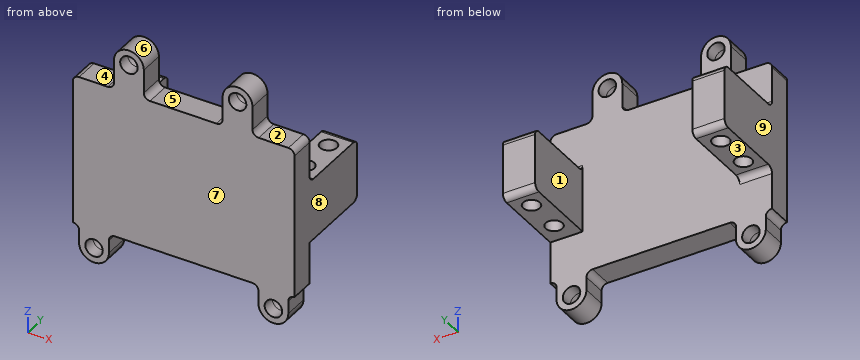
```python
from build123d import *
from build123d.topology import SkipClean

# Parameters (mm, degrees)
SKETCH1_W           = 54.4
SKETCH1_H           = 38.8
BOSS_EXTRUDE1_DEPTH = 3.175
SKETCH2_W           = 7
SKETCH2_H           = 15.875
BOSS_EXTRUDE2_DEPTH = 20
SKETCH3_R           = 3.8354
SKETCH3_R_2         = 2.2479
BOSS_EXTRUDE3_DEPTH = 3.175
LPATTERN1_COUNT     = 2
LPATTERN1_PITCH     = 27.94
SKETCH6_R           = 3.8354
SKETCH6_R_2         = 2.2479
BOSS_EXTRUDE6_DEPTH = 3.175
SKETCH7_R           = 2.150000018
CUT_EXTRUDE1_DEPTH  = 15.875
BOSS_EXTRUDE7_DEPTH = 1.2948
SKETCH11_R          = 2.2479
BOSS_EXTRUDE8_DEPTH = 3.175
FILLET1_R           = 1.5875


with BuildPart() as part:
    # Sketch1 → Boss-Extrude1 (new body)
    with BuildSketch(Plane(origin=(0, 0, 0), x_dir=(1, 0, 0), z_dir=(0, 1, 0))):
        with Locations((27.2, 19.4)):
            Rectangle(SKETCH1_W, SKETCH1_H)
    extrude(amount=BOSS_EXTRUDE1_DEPTH)

    # Sketch2 → Boss-Extrude2 (add)
    with BuildSketch(Plane(origin=(0, 3.175, 0), x_dir=(1, 0, 0), z_dir=(0, 1, 0))):
        with Locations((3.5, 20.0625)):
            Rectangle(SKETCH2_W, SKETCH2_H)
    boss_extrude2 = extrude(amount=BOSS_EXTRUDE2_DEPTH)

    # Mirror1: Boss-Extrude2 across plane
    add(boss_extrude2.mirror(Plane.ZY.offset(-27.2)))

    # Sketch3 → Boss-Extrude3 (add)
    # profile 1 of 2: a face of its own
    with BuildSketch(Plane(origin=(0, 3.175, 0), x_dir=(1, 0, 0), z_dir=(0, 1, 0))):
        with Locations((13.109999942, -7.608)):
            Circle(SKETCH3_R)
        with Locations(Location((13.109999942, -7.608, 0), (0, 0, 270))):
            Circle(SKETCH3_R_2, mode=Mode.SUBTRACT)
    # profile 2 of 2: a face of its own
    with BuildSketch(Plane(origin=(0, 3.175, 0), x_dir=(1, 0, 0), z_dir=(0, 1, 0))):
        with BuildLine():
            Line((9.274599942, 0), (9.274599942, -7.608))
            ThreePointArc((9.274599942, -7.608), (13.109999942, -3.7726), (16.945399942, -7.608))
            Line((16.945399942, -7.608), (16.945399942, 0))
            Line((16.945399942, 0), (9.274599942, 0))
        make_face()
    boss_extrude3 = extrude(amount=-BOSS_EXTRUDE3_DEPTH)

    # LPattern1: Boss-Extrude3 ×2
    with Locations(*[(i * LPATTERN1_PITCH, 0, 0) for i in range(1, LPATTERN1_COUNT)]):
        add(boss_extrude3)

    # Sketch6 → Boss-Extrude6 (add)
    # profile 1 of 2: a face of its own
    with BuildSketch(Plane(origin=(0, 3.175, 0), x_dir=(1, 0, 0), z_dir=(0, 1, 0))):
        with Locations((4.1402, 43.7)):
            Circle(SKETCH6_R)
        with Locations(Location((4.1402, 43.7, 0), (0, 0, 270))):
            Circle(SKETCH6_R_2, mode=Mode.SUBTRACT)
    # profile 2 of 2: a face of its own
    with BuildSketch(Plane(origin=(0, 3.175, 0), x_dir=(1, 0, 0), z_dir=(0, 1, 0))):
        with BuildLine():
            ThreePointArc((7.9756, 43.7), (4.1402, 39.8646), (0.3048, 43.7))
            Line((0.3048, 43.7), (0.3048, 38.8))
            Line((0.3048, 38.8), (7.9756, 38.8))
            Line((7.9756, 38.8), (7.9756, 43.7))
        make_face()
    boss_extrude6 = extrude(amount=-BOSS_EXTRUDE6_DEPTH)

    # Mirror3: Boss-Extrude6 across plane
    add(boss_extrude6.mirror(Plane.ZY.offset(-27.2)))

    # Sketch7 → Cut-Extrude1 (cut)
    with BuildSketch(Plane(origin=(0, 0, -28), x_dir=(-1, 0, 0), z_dir=(0, 0, -1))):
        with Locations((-2.852600116, 17.925)):
            Circle(SKETCH7_R)
        with Locations((-2.852600116, 8.425)):
            Circle(SKETCH7_R)
    cut_extrude1 = extrude(amount=-CUT_EXTRUDE1_DEPTH, mode=Mode.SUBTRACT)

    # Sketch9 → Boss-Extrude7 (add)
    with BuildSketch(Plane.ZY):
        Polygon((-38.8, 0), (-38.8, 3.175), (-28, 3.175), (-28, 23.175), (-12.125, 23.175), (-12.125, 3.175), (0, 3.175), (0, 0), align=None)
    boss_extrude7 = extrude(amount=BOSS_EXTRUDE7_DEPTH)

    # Mirror4: Boss-Extrude7 across plane
    add(boss_extrude7.mirror(Plane.ZY.offset(-27.2)))

    # Mirror5: Cut-Extrude1 across plane
    add(cut_extrude1.mirror(Plane.ZY.offset(-27.2)), mode=Mode.SUBTRACT)

    # Sketch11 → Boss-Extrude8 (add)
    with SkipClean():  # the faces are left unmerged after this step: merging them gives an invalid solid
        with BuildSketch(Plane.XZ):
            with BuildLine():
                Line((0.3048, -38.8), (0.3048, -43.7))
                ThreePointArc((0.3048, -43.7), (4.1402, -47.5354), (7.9756, -43.7))
                Line((7.9756, -43.7), (7.9756, -38.8))
                Line((7.9756, -38.8), (46.4244, -38.8))
                Line((46.4244, -38.8), (46.4244, -43.7))
                ThreePointArc((46.4244, -43.7), (50.2598, -47.5354), (54.0952, -43.7))
                Line((54.0952, -43.7), (54.0952, -38.8))
                Line((54.0952, -38.8), (55.6948, -38.8))
                Line((55.6948, -38.8), (55.6948, 0))
                Line((55.6948, 0), (44.885399942, 0))
                Line((44.885399942, 0), (44.885399942, 7.608))
                ThreePointArc((44.885399942, 7.608), (41.049999942, 11.4434), (37.214599942, 7.608))
                Line((37.214599942, 7.608), (37.214599942, 0))
                Line((37.214599942, 0), (16.945399942, 0))
                Line((16.945399942, 0), (16.945399942, 7.608))
                ThreePointArc((16.945399942, 7.608), (13.109999942, 11.4434), (9.274599942, 7.608))
                Line((9.274599942, 7.608), (9.274599942, 0))
                Line((9.274599942, 0), (-1.2948, 0))
                Line((-1.2948, 0), (-1.2948, -38.8))
                Line((-1.2948, -38.8), (0.3048, -38.8))
            make_face()
            with Locations(Location((4.1402, -43.7, 0), (0, 0, 90))):
                Circle(SKETCH11_R, mode=Mode.SUBTRACT)
            with Locations(Location((50.2598, -43.7, 0), (0, 0, 90))):
                Circle(SKETCH11_R, mode=Mode.SUBTRACT)
            with Locations(Location((41.049999942, 7.608, 0), (0, 0, 90))):
                Circle(SKETCH11_R, mode=Mode.SUBTRACT)
            with Locations(Location((13.109999942, 7.608, 0), (0, 0, 90))):
                Circle(SKETCH11_R, mode=Mode.SUBTRACT)
        extrude(amount=BOSS_EXTRUDE8_DEPTH)
    add(part.part.scale(1), mode=Mode.REPLACE)  # the faces are merged on a copy

    # Fillet1
    fillet1_edges = [part.edges().sort_by_distance(p)[0] for p in [
        (-1.2948, 0, 0),
        (55.6948, 0, 0),
        (2.8526, 3.175, -12.125),
        (2.8526, 3.175, -28),
        (2.8526, 23.175, -12.125),
        (2.8526, 23.175, -28),
        (51.5474, 23.175, -28),
        (51.5474, 23.175, -12.125),
        (51.5474, 3.175, -12.125),
        (16.945399942, 0, 0),
        (9.274599942, 0, 0),
        (44.885399942, 0, 0),
        (37.214599942, 0, 0),
        (0.3048, 0, -38.8),
        (7.9756, 0, -38.8),
        (46.4244, 0, -38.8),
        (54.0952, 0, -38.8),
    ]]
    fillet(fillet1_edges, radius=FILLET1_R)


solid = part.part
```
Read the model definition and answer for the solid it produces. Units are mm, in the model's axes. Face numbers are marked on the shaded views. A direction names the side the tool comes from. Give positions to 0.01 mm unless a question says otherwise; leave off trailing zeros. Loops run counter-clockwise (first coordinate to the right, second up) from the corner with the lowest first, then second, coordinate; pieces in that order, holes last.
Item 1: Find the intervals of material crossed by line 1 along Z through (x, y) = (13.11, 1.3); line 2 along X through (y, z) = (20.75, -20.5); line 3 along X through (y, z) = (0.25, 7.5), in increasing order.
Item 2: The mould has two halves that part along X. Classify the marked faces 6, 7, 8 and 9: released by +X, released by -X, zero draft, split by the parting line, or undercut.
Item 3: The part is cut by section C-C (x = 13.11). Write down the section's boundary in (y, z) (3 decimals).
Item 4: The part is cut by section B-B (y = 19.25). Write down the section's boundary in (x, z) (3 decimals), and give its area (3 significant figures).
Item 5: Each of these flat-tipped pins is pushed along its axis until it touches: pin 1 Ø2.5 at (x, y) = (52, 16.5) entering from -Z; pin 2 Ø3.5 at (x, y) = (51.55, 8.43) entering from -Z; pin 3 Ø4 at (x, y) = (51, 16.5) entering from +Z (3 decimals); pin 4 Ø1 at (y, z) = (0.5, -43) entering from -X. Where does it stop, or does it pass through?
Item 6: For the marked faces 1, 2, 3, 4 and 5, determine the directions among +Z, -Z, +X, -X, +Y, -Y from which every point of the face is accessible in a straight line to the end or side of a thin tool.
Item 7: The part is cut by section D-D (y = -1.5). Give the number of separate pieces and of enclosed holes in the cut face, and give its area (3 significant figures).
Item 8: The part is cut by section A-A (z = 4). Write down the section's boundary in (x, y) (3 decimals).
Taken from the geometry:
1. line 1: z = -38.8 to 5.36, 9.86 to 11.44
1. line 2: x = -1.29 to 7, 47.4 to 55.69
1. line 3: x = 9.27 to 10.86, 15.36 to 16.95, 37.21 to 38.8, 43.3 to 44.89
2. face 6: undercut
2. face 7: zero draft
2. face 8: released by +X
2. face 9: released by -X
3. outline: (-3.175, -38.8) - (3.175, -38.8) - (3.175, 5.36) - (-3.175, 5.36) - close; (-3.175, 9.856) - (3.175, 9.856) - (3.175, 11.443) - (-3.175, 11.443) - close
4. outline: (-1.295, -28) - (1.159, -28) - (1.159, -12.125) - (-1.295, -12.125) - close; (4.546, -28) - (7, -28) - (7, -12.125) - (4.546, -12.125) - close; (47.4, -28) - (49.854, -28) - (49.854, -12.125) - (47.4, -12.125) - close; (53.241, -28) - (55.695, -28) - (55.695, -12.125) - (53.241, -12.125) - close
4. area: 156 mm2
5. pin 1: stops at z = -28
5. pin 2: passes through
5. pin 3: stops at z = -12.125
5. pin 4: stops at x = 0.3
6. face 1: +Z, -Z, +Y
6. face 2: +Z, +X, +Y, -Y
6. face 3: -Z, +X, -X, +Y
6. face 4: +Z, -X, +Y, -Y
6. face 5: +Z, +Y, -Y
7. separate pieces: 1
7. enclosed holes: 4
7. area: 2,440 mm2
8. outline: (9.275, -3.175) - (16.945, -3.175) - (16.945, 3.175) - (9.275, 3.175) - close; (37.215, -3.175) - (44.885, -3.175) - (44.885, 3.175) - (37.215, 3.175) - close
